Read the model definition and answer for the solid it produces. Units are mm, in the model's axes. Face numbers are marked on the shaded views. Coordinates: 2 decimals unless noted, no trailing zeros. Write each loop counter-clockwise with the first axis right and the second up, starting at its lowest first coordinate (ties: lowest second). Pieces come first, ordered by that corner, then holes. Notation, with made-up numbers: (41, 7) -> (84, 7) arc R19 ccw to (84, 15) -> close; hole circle Ø5 at (7.25, 88.25). An arc over 180 degrees is marked (long way). Answer as a JSON object with one key per item and string values. Group by question number.
(1) Find section C-C (y = 43.5). Give the vertices of the cut face in (x, z).
(2) Straight lines are drawn through the part: L1, parallel to X at y = -27.5, z = 78; L2, parallel to Y at x = 6, z = 27; L3, parallel to Z at x = -46, y = 32. For each, find the intervals that lie inside material, in ascending order.
(3) Find section A-A (z = 68). Give the vertices of the cut face in (x, y).
(4) Find section B-B (x = 30.5). Give the vertices of the cut face in (y, z).
(5) For a pull along Y with two mould halves and no side action, classify the marked faces 1, 2, 3 and 4 as +Y half, -Y half, draft (parallel to the pull), parting line (faces both ways), or undercut.
from build123d import *

# Parameters (mm, degrees)
F0_W        = 102.4
F0_H        = 85.6
F1_DEPTH    = 89.75
F2_T        = 2.54
F3_T1_DEPTH = 117.69


# Not quite as in the source:
# - a fillet or chamfer that OpenCascade refuses, or shapes differently, is made with other operations: its cross-section is extruded or revolved along the edge and cut away or added


with BuildPart() as f1:
    # F0 (on Top) → F1 (new body)
    with BuildSketch(Plane.XY):
        with Locations((0.6768562123, 7.1260996301)):
            Rectangle(F0_W, F0_H)
    extrude(amount=F1_DEPTH)

    # F2
    f2_openings = [f1.faces().sort_by_distance(p)[0] for p in [
        (0.676856, 7.1261, 89.75),
    ]]
    offset(amount=F2_T, openings=f2_openings, kind=Kind.INTERSECTION)

    # F3: fillet of radius 5.08 on 4 edges, made by hand

    # F3_s2 → F3_t1 (cut)
    with BuildSketch(Plane.XY.offset(-15.24)):
        with BuildLine():
            ThreePointArc((49.3368562123, 52.4660996301), (52.9289586607, 50.9782020785), (54.4168562123, 47.3860996301))
            Line((54.4168562123, 47.3860996301), (54.4168562123, 52.4660996301))
            Line((54.4168562123, 52.4660996301), (49.3368562123, 52.4660996301))
        make_face()
        with BuildLine():
            ThreePointArc((-47.9831437877, 52.4660996301), (-51.5752462361, 50.9782020785), (-53.0631437877, 47.3860996301))
            Line((-53.0631437877, 47.3860996301), (-53.0631437877, 52.4660996301))
            Line((-53.0631437877, 52.4660996301), (-47.9831437877, 52.4660996301))
        make_face()
        with BuildLine():
            ThreePointArc((-53.0631437877, -33.1339003699), (-51.5752462361, -36.7260028183), (-47.9831437877, -38.2139003699))
            Line((-47.9831437877, -38.2139003699), (-53.0631437877, -38.2139003699))
            Line((-53.0631437877, -38.2139003699), (-53.0631437877, -33.1339003699))
        make_face()
        with BuildLine():
            ThreePointArc((49.3368562123, -38.2139003699), (52.9289586607, -36.7260028183), (54.4168562123, -33.1339003699))
            Line((54.4168562123, -33.1339003699), (54.4168562123, -38.2139003699))
            Line((54.4168562123, -38.2139003699), (49.3368562123, -38.2139003699))
        make_face()
    extrude(amount=F3_T1_DEPTH, mode=Mode.SUBTRACT)


solid = f1.part
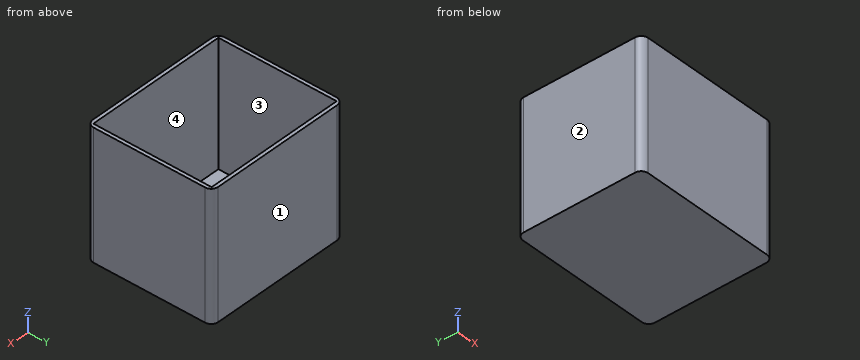
Results below:
{
 "1": {"outline": "(-53.06, -2.54) -> (54.42, -2.54) -> (54.42, 89.75) -> (51.88, 89.75) -> (51.88, 0) -> (-50.52, 0) -> (-50.52, 89.75) -> (-53.06, 89.75) -> close"},
 "2": {"L1": "x = -53.06 to -50.52, 51.88 to 54.42", "L2": "y = -38.21 to -35.67, 49.93 to 52.47", "L3": "z = -2.54 to 0"},
 "3": {"outline": "(-53.06, -33.13) arc R5.08 ccw to (-47.98, -38.21) -> (49.34, -38.21) arc R5.08 ccw to (54.42, -33.13) -> (54.42, 47.39) arc R5.08 ccw to (49.34, 52.47) -> (-47.98, 52.47) arc R5.08 ccw to (-53.06, 47.39) -> close; hole (-50.52, -35.67) -> (51.88, -35.67) -> (51.88, 49.93) -> (-50.52, 49.93) -> close"},
 "4": {"outline": "(-38.21, -2.54) -> (52.47, -2.54) -> (52.47, 89.75) -> (49.93, 89.75) -> (49.93, 0) -> (-35.67, 0) -> (-35.67, 89.75) -> (-38.21, 89.75) -> close"},
 "5": {"face 1": "+Y half", "face 2": "draft", "face 3": "undercut", "face 4": "undercut"}
}
